Geometry: final body of the model. Coordinates: model frame, mm. A direction names the side the tool comes from. Coordinates: 2 decimals unless noted, no trailing zeros. Write each loop counter-clockwise with the first axis right and the second up, starting at its lowest first coordinate (ties: lowest second). Pieces come first, ordered by that corner, then holes.
from build123d import *

# Parameters (mm, degrees)
SKETCH1_R           = 0.125
BOSS_EXTRUDE1_DEPTH = 1
SCALE1_SCALE        = 25.399986
BOSS_EXTRUDE2_START = 19.05
SKETCH2_W           = 126.99993
SKETCH2_H           = 19.0499895
SKETCH2_R           = 3.17499825
BOSS_EXTRUDE2_DEPTH = 19.05


with BuildPart() as part:
    # Sketch1 → Boss-Extrude1 (new body)
    with BuildSketch(Plane.XY):
        Polygon((6.53415074, 29.25), (8.449452651, 22.685482615), (0, 0), (3, 0), (9.03415074, 20.681484839), (15.06830148, 0), (18.06830148, 0), (9.618848829, 22.685482615), (11.53415074, 29.25), (11.53415074, 30), (6.53415074, 30), align=None)
        Polygon((7.173823534, 29.25), (10.894477946, 29.25), (9.03415074, 24.25530718), align=None, mode=Mode.SUBTRACT)
        with Locations((7.03415074, 29.625)):
            Circle(SKETCH1_R, mode=Mode.SUBTRACT)
        with Locations((11.03415074, 29.625)):
            Circle(SKETCH1_R, mode=Mode.SUBTRACT)
    extrude(amount=BOSS_EXTRUDE1_DEPTH)


with BuildPart() as part_1:
    # Scale1: scaled about (9.03415074, 11.863251785, 0.5)
    add(part.part.scale(SCALE1_SCALE).moved(Location((-220.433151578, -289.463177468, -12.199993))))

    # Sketch2 → Boss-Extrude2 (add)
    with BuildSketch(Plane(origin=(0, 0, -12.199993), x_dir=(-1, 0, 0), z_dir=(0, 0, -1)).offset(BOSS_EXTRUDE2_START)):
        with Locations((-9.03415074, 463.011407788)):
            Rectangle(SKETCH2_W, SKETCH2_H)
        with Locations((-59.83412274, 463.011407788)):
            Circle(SKETCH2_R, mode=Mode.SUBTRACT)
        with Locations((41.76582126, 463.011407788)):
            Circle(SKETCH2_R, mode=Mode.SUBTRACT)
    extrude(amount=-BOSS_EXTRUDE2_DEPTH)


solid = part_1.part
Item 1: Section A-A, the plane y = -54.5. Output: boundary loops of the cut face in (x, z).
Derived:
outline: (-132.92, -12.2) - (-75.68, -12.2) - (-75.68, 13.2) - (-132.92, 13.2) - close; (93.75, -12.2) - (150.99, -12.2) - (150.99, 13.2) - (93.75, 13.2) - close
Item 2: Section B-B, the plane z = 4. State how many separate pieces and enclosed holes the cut face has, plus the area to 3 significant figures.
Derived:
separate pieces: 1
enclosed holes: 3
area: 69,700 mm2
Item 3: Section C-C, the plane y = 136.5. Output: boundary loops of the cut face in (x, z).
Derived:
outline: (-61.78, -12.2) - (-19.95, -12.2) - (-19.95, 13.2) - (-61.78, 13.2) - close; (38.02, -12.2) - (79.85, -12.2) - (79.85, 13.2) - (38.02, 13.2) - close
Item 4: Pin query (flat end, axial travel): pin 1 (10 mm diameter, centred on y = -186, z = -3, fed in from -X); pin 2 (10 mm diameter, centred on x = 21.5, z = -24, fed in from -Y); pin 3 (9.5 mm diameter, centred on y = 465.5, z = -1.5, fed in from -X); pin 4 (5.5 mm diameter, centred on x = -41.77, y = 463.01, fed in from -Z). Return the tip coordinate at first contact, or that it passes through.
Derived:
pin 1: stops at x = -183.76
pin 2: stops at y = 453.49
pin 3: stops at x = -54.47
pin 4: passes through
Item 5: Material intervals for probe 1 along Z at (x, y) = (81, 70); probe 2 along X at (y, z) = (-9.5, 6); probe 3 along X at (y, z) = (-100, -4.5), sorted ascending.
Derived:
probe 1: z = -12.2 to 13.2
probe 2: x = -116.16 to -62.55, 80.62 to 134.23
probe 3: x = -149.87 to -88.95, 107.02 to 167.93
Item 6: Set-up query: faces 1 (the flat face through (-30.48, 371.28, 0.32)), 2 (the flat face through (32.99, 390.94, 0.32)), 3 (the flat face through (-54.466, 463, -9)). Return all of +Z, -Z, +X, -X, +Y, -Y with unobstructed straight access to the full face (end or side cutting, diameter ignored); none if empty.
Derived:
face 1: +Z, -Z, -X
face 2: +Z, -Z
face 3: +Z, -Z, -X, +Y
Item 7: Section D-D, the plane x = 127.5. Output: boundary loops of the cut face in (y, z).
Derived:
outline: (-170.18, -12.2) - (8.56, -12.2) - (8.56, 13.2) - (-170.18, 13.2) - close
Item 8: Pull-direction query (X, two-part tool) for faces 4 (the flat face through (132.7, -5.4, 0.3)), 5 (the flat face through (10, 453.486, -9)), 6 (the flat face through (76, 29, -12.2)); classes: released by +X, released by -X, zero draft, split by the parting line, or undercut.
Derived:
face 4: released by +X
face 5: undercut
face 6: zero draft
